from build123d import *

# Parameters (mm, degrees)
F1_DEPTH    = 20
F2_T1_DEPTH = 20
F3_T1_DEPTH = 32.2692705553
F5_R        = 5


# Not quite as in the source:
# - a fillet or chamfer that OpenCascade refuses, or shapes differently, is made with other operations: its cross-section is extruded or revolved along the edge and cut away or added


with BuildPart() as f1:
    # F0 (on Top) → F1 (new body)
    with BuildSketch(Plane.XY):
        Polygon((0, 2.0882352941), (0, 0), (10, 0), (44, 6.5), (44, 13.5), (10, 20), (2, 20), (0, 20), (0, 17.9117647059), (10, 16), (41.3846153846, 10), (10, 4), align=None)
        with BuildLine():
            Line((0, 20), (2, 20))
            ThreePointArc((2, 20), (1, 21), (0, 20))
        make_face()
    extrude(amount=-F1_DEPTH)

    # F2: fillet of radius 1 on 1 edges, made by hand

    # F2_s2 → F2_t1 (join)
    with BuildSketch(Plane.XY.offset(-20)):
        with BuildLine():
            ThreePointArc((36.2468915209, 10.9822119151), (37.0591157136, 10), (36.2468915209, 9.0177880849))
            Line((36.2468915209, 9.0177880849), (41.3846153846, 10))
            Line((41.3846153846, 10), (36.2468915209, 10.9822119151))
        make_face()
    extrude(amount=F2_T1_DEPTH)

    # F3: fillet of radius 3 on 2 edges, made by hand

    # F3_s2 → F3_t1 (cut)
    with BuildSketch(Plane.XY.offset(-26.1346352777)):
        with BuildLine():
            ThreePointArc((0, 20), (0.7936912123, 18.3364871524), (2.4102047458, 17.4509902692))
            Line((2.4102047458, 17.4509902692), (2.3989381974, 17.3920575543))
            Line((2.3989381974, 17.3920575543), (-0.0112665484, 17.852831991))
            Line((-0.0112665484, 17.852831991), (-0.06, 17.9117647059))
            ThreePointArc((-0.06, 17.9117647059), (-0.06, 18.9558823529), (-0.0594706434, 19.9920474797))
            Line((-0.0594706434, 19.9920474797), (0, 20))
        make_face()
        with BuildLine():
            ThreePointArc((0, 0), (0.7936912123, 1.6635128476), (2.4102047458, 2.5490097308))
            Line((2.4102047458, 2.5490097308), (2.3989381974, 2.6079424457))
            Line((2.3989381974, 2.6079424457), (-0.0112665484, 2.147168009))
            Line((-0.0112665484, 2.147168009), (-0.06, 2.0882352941))
            ThreePointArc((-0.06, 2.0882352941), (-0.06, 1.0441176471), (-0.0594706434, 0.0079525203))
            Line((-0.0594706434, 0.0079525203), (0, 0))
        make_face()
    extrude(amount=F3_T1_DEPTH, mode=Mode.SUBTRACT)

    # F4: F1 across face


with BuildPart() as f1_1:
    add(f1.part)
    add(f1.part.mirror(Plane(origin=(44, 10, -10), x_dir=(0, 1, 0), z_dir=(1, 0, 0))))

    # F5
    f5_edges = [f1_1.edges().sort_by_distance(p)[0] for p in [
        (44, 13.5, -10),
        (44, 6.5, -10),
    ]]
    fillet(f5_edges, radius=F5_R)


solid = f1_1.part
Input: part model. Units: mm. Frame: model coordinates. A direction names the side the tool comes from. Round coordinates to 2 decimals unless told otherwise and drop trailing zeros. Order: outer loops, then holes, each group sorted by start corner. A loop starts at its lowest first (then second) coordinate and runs counter-clockwise, first axis right, second up. Notation, with made-up numbers: (79, -27) - (113, -27) arc R6 ccw to (113, -21) - close; hole circle Ø9 at (38, 3.25). An arc over 180 degrees is marked (long way). Answer as a JSON object with one key per item and string values. Group by question number.
(1) Material intervals for probe 1 along Y at (x, z) = (78, -13.5); probe 2 along Y at (x, z) = (80, -7.5); probe 3 along Y at (x, z) = (43, -17.75), sorted ascending. Write a range as from..to.
(2) Cut plane B-B (x = 1). Return loops of the section in (y, z), then the cut area to 3 significant figures.
(3) Pin query (flat end, axial travel): P1, Ø4, axis at x = 47.5, z = -8, coming from the -Y side; P2, Ø2.5, axis at x = 4.5, z = -10, coming from the +Y side; P3, Ø4, axis at x = 69.5, z = -12, coming from the -Y side. Return the tip coordinate at first contact, or that it passes through.
(4) Reachability of faces 1 (the face through (0.776, 18.356, -10.14)), 2 (the face through (26.299, 3.116, -9.86)), 3 (the face through (61.238, 16.796, -9.86)) from +Z, -Z, +X, -X, +Y, -Y: full face, straight path, thin tool, end or side. Return the list, or none.
(5) Draft query along Y for faces 4 (the face through (0.776, 1.644, -10.14)), 5 (the face through (87.224, 1.644, -10.14)), 6 (the face through (45, 11, -20)), 7 (the face through (26.762, 16.796, -9.86)). Return one class per face: released by +Y, released by -Y, zero draft, split by the parting line, or undercut.
(6) Cut plane A-A (z = -15.5). Return loops of the section in (x, y).
(7) Cut plane C-C (y = 15). Return loops of the section in (x, z).
Here are the results:
{
 "1": {"probe 1": "y = 0..4, 16..20", "probe 2": "y = 0..3.62, 16.38..20", "probe 3": "y = 6.31..13.69"},
 "2": {"outline": "(0, -20) - (1.86, -20) - (1.86, 0) - (0, 0) - close; (18.14, -20) - (21, -20) - (21, 0) - (18.14, 0) - close", "area": "94.5 mm^2"},
 "3": {"P1": "stops at y = 5.45", "P2": "stops at y = 20", "P3": "stops at y = 1.24"},
 "4": {"face 1": "+Z, -Z, -X", "face 2": "+Z, -Z, -Y", "face 3": "+Z, -Z, +Y"},
 "5": {"face 4": "undercut", "face 5": "undercut", "face 6": "zero draft", "face 7": "released by +Y"},
 "6": {"outline": "(0, 0) - (10, 0) - (43.06, 6.32) arc R5 cw to (44.94, 6.32) - (78, 0) - (88, 0) arc R3 ccw to (85.59, 2.55) - (51.75, 9.02) arc R1 cw to (51.75, 10.98) - (85.59, 17.45) arc R3 ccw to (88, 20) arc R1 ccw to (86, 20) - (78, 20) - (44.94, 13.68) arc R5 cw to (43.06, 13.68) - (10, 20) - (2, 20) arc R1 ccw to (0, 20) arc R3 ccw to (2.41, 17.45) - (36.25, 10.98) arc R1 cw to (36.25, 9.02) - (2.41, 2.55) arc R3 ccw to start"},
 "7": {"outline": "(15.23, -20) - (36.15, -20) - (36.15, 0) - (15.23, 0) - close; (51.85, -20) - (72.77, -20) - (72.77, 0) - (51.85, 0) - close"}
}
